Verification items for the finished model (mm, model axes). Coordinates: 2 decimals unless noted, no trailing zeros. Write each loop counter-clockwise with the first axis right and the second up, starting at its lowest first coordinate (ties: lowest second). Pieces come first, ordered by that corner, then holes. Notation, with made-up numbers: (28.5, 36) - (82.5, 36) arc R23 ccw to (82.5, 52) - close; hole circle Ø9 at (-10.75, 7.25). An arc over 180 degrees is marked (long way). Answer as CSV lines item,"result". Start each with the question number.
```python
from build123d import *

# Parameters (mm, degrees)
SKETCH2_R           = 38.5
BOSS_EXTRUDE4_DEPTH = 1.5
BOSS_EXTRUDE5_DEPTH = 1.5
SKETCH4_R           = 1.6
CUT_EXTRUDE1_DEPTH  = 1.5
FILLET1_R           = 10


with BuildPart() as part:
    # Sketch2 → Boss-Extrude4 (new body)
    with BuildSketch(Plane(origin=(0, 0, 0), x_dir=(1, 0, 0), z_dir=(0, 1, 0))):
        with BuildLine():
            Line((-60, 32), (-28.722813233, 32))
            ThreePointArc((-28.722813233, 32), (0, 43), (28.722813233, 32))
            Line((28.722813233, 32), (60, 32))
            Line((60, 32), (60, -32))
            Line((60, -32), (28.722813233, -32))
            ThreePointArc((28.722813233, -32), (0, -43), (-28.722813233, -32))
            Line((-28.722813233, -32), (-60, -32))
            Line((-60, -32), (-60, 32))
        make_face()
        Circle(SKETCH2_R, mode=Mode.SUBTRACT)
    extrude(amount=BOSS_EXTRUDE4_DEPTH)

    # Sketch3 → Boss-Extrude5 (add)
    with BuildSketch(Plane(origin=(0, 1.5, 0), x_dir=(1, 0, 0), z_dir=(0, 1, 0))):
        Polygon((60, 32), (60, 33), (22.967632109, 33), (40.759186936, 20.496414307), (60, 20.496414307), align=None)
        Polygon((60, -20.496414307), (60, -32), (60, -33), (22.967632109, -33), (40.759186936, -20.496414307), align=None)
        Polygon((-60, -32), (-60, -33), (-22.967632109, -33), (-40.759186936, -20.496414307), (-60, -20.496414307), align=None)
        Polygon((-60, 20.496414307), (-60, 32), (-60, 33), (-22.967632109, 33), (-40.759186936, 20.496414307), align=None)
    extrude(amount=-BOSS_EXTRUDE5_DEPTH)

    # Sketch4 → Cut-Extrude1 (cut)
    with BuildSketch(Plane(origin=(0, 1.5, 0), x_dir=(1, 0, 0), z_dir=(0, 1, 0))):
        with Locations((40, 28)):
            Circle(SKETCH4_R)
        with Locations((40, -28)):
            Circle(SKETCH4_R)
        with Locations((-40, -28)):
            Circle(SKETCH4_R)
        with Locations((-40, 28)):
            Circle(SKETCH4_R)
    extrude(amount=-CUT_EXTRUDE1_DEPTH, mode=Mode.SUBTRACT)

    # Fillet1
    fillet1_edges = [part.edges().sort_by_distance(p)[0] for p in [
        (60, 0.75, -33),
        (60, 0.75, 33),
        (-60, 0.75, 33),
        (-60, 0.75, -33),
    ]]
    fillet(fillet1_edges, radius=FILLET1_R)


solid = part.part
```
1. Cross-section at D-D (x = 12). Record the cut outline in (y, z).
2. Draft check along Z on faces 1 (the face through (39.792, 0.76, -29.586)), 2 (the face through (57.15, 0.74, 29.99)), 3 (the face through (-30.55, 0.74, 23.43)), 4 (the face through (-56.99, 0.74, -30.15)). Enter one of: pulls with the +Z half, pulls with the -Z half, needs draft (parallel to the pull), parting line crosses it, or undercut.
3. Scan lines: line 1 along Z through (x, y) = (40, 0.55); line 2 along X through (y, z) = (0.65, -28); line 3 along X through (y, z) = (1, 3). Record each from-to range of solid material in increasing order. Write a range as from..to.
4. Cross-section at B-B (y = 0.35). Record the cut outline in (x, z).
5. Depth check by flat-ended pin: P1, Ø1.9, axis at x = -40, z = -28, coming from the +Y side; P2, Ø0.8, axis at x = 35.5, y = 0.5, coming from the +Z side; P3, Ø0.8, axis at x = -34.5, y = 0.5, coming from the -Z side. Enter the tip coordinate at first touch or a pass-through.
6. Cross-section at C-C (z = 0). Record the cut outline in (x, y), and give its area (3 significant figures).
7. Cross-section at A-A (x = -40). Record the cut outline in (y, z).
Completed:
1,outline,"(0, -41.29) - (1.5, -41.29) - (1.5, -36.58) - (0, -36.58) - close; (0, 36.58) - (1.5, 36.58) - (1.5, 41.29) - (0, 41.29) - close"
2,face 1,"undercut"
2,face 2,"pulls with the +Z half"
2,face 3,"undercut"
2,face 4,"pulls with the -Z half"
3,line 1,"z = -33..-29.6, -26.4..26.4, 29.6..33"
3,line 2,"x = -58.66..-41.6, -38.4..-26.42, 26.42..38.4, 41.6..58.66"
3,line 3,"x = -60..-38.38, 38.38..60"
4,outline,"(-60, -23) arc R10 ccw to (-50, -33) - (-27.57, -33) arc R43 ccw to (27.57, -33) - (50, -33) arc R10 ccw to (60, -23) - (60, 23) arc R10 ccw to (50, 33) - (27.57, 33) arc R43 ccw to (-27.57, 33) - (-50, 33) arc R10 ccw to (-60, 23) - close; hole circle Ø3.2 at (-40, -28); hole circle Ø3.2 at (-40, 28); hole circle Ø77 at (0, 0); hole circle Ø3.2 at (40, -28); hole circle Ø3.2 at (40, 28)"
5,P1,"passes through"
5,P2,"stops at z = 33"
5,P3,"stops at z = -33"
6,outline,"(-60, 0) - (-38.5, 0) - (-38.5, 1.5) - (-60, 1.5) - close; (38.5, 0) - (60, 0) - (60, 1.5) - (38.5, 1.5) - close"
6,area,"64.5 mm2"
7,outline,"(0, -33) - (1.5, -33) - (1.5, -29.6) - (0, -29.6) - close; (0, -26.4) - (1.5, -26.4) - (1.5, 26.4) - (0, 26.4) - close; (0, 29.6) - (1.5, 29.6) - (1.5, 33) - (0, 33) - close"
